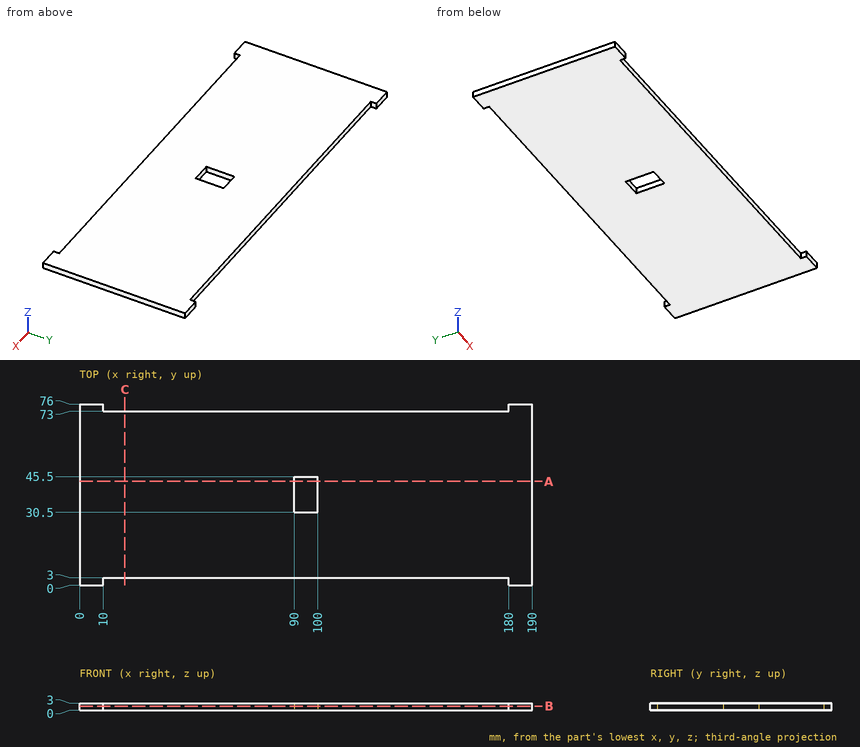
Study the drawing (mm; zero at the part's minimum x, y, z) and answer. Coordinates: 2 decimals unless noted, no trailing zeros. Order: outer loops, then holes, each group sorted by start corner. A loop starts at its lowest first (then second) coordinate and runs counter-clockwise, first axis right, second up. Notation, with made-up numbers: M 69.25,-26 L 106.25,-26 A28 ccw 106.25,-5 Z; hole C 89,84.25 d11. An arc over 180 degrees is marked long. Use CSV: the item, a comma, the result in double quotes.
Q1. Straight lines are drawn through the part: L1, parallel to X at y = 36, z = 2.1; L2, parallel to Y at x = 98, z = 2.2; L3, parallel to Y at x = 11.5, z = 0.6. For each, find the intervals that lie inside material, in ascending order.
Here are the results:
L1,"0 to 90, 100 to 190"
L2,"3 to 30.5, 45.5 to 73"
L3,"3 to 73"
Q2. Section B-B (z = 1.8) is taken. Determine the outline of the cut face in (x, y).
Here are the results:
outline,"M 0,0 L 10,0 L 10,3 L 180,3 L 180,0 L 190,0 L 190,76 L 180,76 L 180,73 L 10,73 L 10,76 L 0,76 Z; hole M 90,30.5 L 100,30.5 L 100,45.5 L 90,45.5 Z"
Q3. Given pin 1 Ø1.5 at (x, z) = (62, 1.5) entering from -Y; pin 2 Ø1.5 at (x, z) = (114.5, 1) entering from +Y, each flat-ended and moving along its own axis, determine where each tip first touches the part or whether it passes through.
Here are the results:
pin 1,"y = 3"
pin 2,"y = 73"
Q4. Section A-A (y = 43.5) is taken. Determine the outline of the cut face in (x, z).
Here are the results:
outline,"M 0,0 L 90,0 L 90,3 L 0,3 Z; M 100,0 L 190,0 L 190,3 L 100,3 Z"
Q5. Section C-C (x = 19) is taken. Determine the outline of the cut face in (y, z), then the cut area to 3 significant figures.
Here are the results:
outline,"M 3,0 L 73,0 L 73,3 L 3,3 Z"
area,"210 mm2"
